```python
from build123d import *

# Parameters (mm, degrees)
BOSS_EXTRUDE1_DEPTH = 35.179
CUT_EXTRUDE2_START  = -5.0038
SKETCH2_R           = 4
CUT_EXTRUDE2_DEPTH  = 5.0038
CUT_EXTRUDE3_START  = -5.674182
CUT_EXTRUDE3_DEPTH  = 5.674182


with BuildPart() as part:
    # Sketch1 → Boss-Extrude1 (new, symmetric)
    with BuildSketch(Plane.XY):
        Polygon((0, 0), (27.178, 0), (27.178, 5.0038), (1.340764169, 5.0038), (-15.645662336, 14.810917915), (-18.147562336, 10.4775), align=None)
    extrude(amount=BOSS_EXTRUDE1_DEPTH, both=True)

    # Sketch2 → Cut-Extrude2 (cut)
    with BuildSketch(Plane.XZ.offset(CUT_EXTRUDE2_START)):
        with Locations(Location((13.462, 0, 0), (0, 0, 270))):
            Circle(SKETCH2_R)
        with BuildLine():
            Line((1.340764169, 35.179), (53.015235831, 35.179))
            Line((53.015235831, 35.179), (53.015235831, -35.179))
            Line((53.015235831, -35.179), (1.340764169, -35.179))
            ThreePointArc((1.340764169, -35.179), (8.255118058, -33.308689777), (13.28379292, -28.207829149))
            Line((13.28379292, -28.207829149), (25.405028751, -6.744829149))
            ThreePointArc((25.405028751, -6.744829149), (27.178, 0), (25.405028751, 6.744829149))
            Line((25.405028751, 6.744829149), (13.28379292, 28.207829149))
            ThreePointArc((13.28379292, 28.207829149), (8.255118058, 33.308689777), (1.340764169, 35.179))
        make_face()
    extrude(amount=CUT_EXTRUDE2_DEPTH, mode=Mode.SUBTRACT)

    # Sketch3 → Cut-Extrude3 (cut)
    with BuildSketch(Plane(origin=(0, 0, 0), x_dir=(0, 0, 1), z_dir=(-0.4999999999999947, -0.8660254037844417, 0)).offset(CUT_EXTRUDE3_START)):
        with BuildLine():
            Line((22.606, 6.928764169), (-22.606, 6.928764169))
            ThreePointArc((-22.606, 6.928764169), (-25.4, 4.134764169), (-22.606, 1.340764169))
            Line((-22.606, 1.340764169), (22.606, 1.340764169))
            ThreePointArc((22.606, 1.340764169), (25.4, 4.134764169), (22.606, 6.928764169))
        make_face()
        with BuildLine():
            Line((-35.179, -1.161135831), (-35.179, 43.071135831))
            Line((-35.179, 43.071135831), (35.179, 43.071135831))
            Line((35.179, 43.071135831), (35.179, -1.161135831))
            ThreePointArc((35.179, -1.161135831), (34.029362855, 4.335697857), (30.773170225, 8.911072784))
            ThreePointArc((30.773170225, 8.911072784), (0, 20.955), (-30.773170225, 8.911072784))
            ThreePointArc((-30.773170225, 8.911072784), (-34.029362855, 4.335697857), (-35.179, -1.161135831))
        make_face()
    extrude(amount=CUT_EXTRUDE3_DEPTH, mode=Mode.SUBTRACT)


solid = part.part
```
Check sheet for the modelled part. Datum: model origin and axes. Units: mm. A direction names the side the tool comes from. Round coordinates to 2 decimals unless told otherwise and drop trailing zeros. Loops run counter-clockwise (first coordinate to the right, second up) from the corner with the lowest first, then second, coordinate; pieces in that order, holes last. Notation, with made-up numbers: (62.5, -22.5) - (76.5, -22.5) arc R27 ccw to (76.5, 13.5) - close; hole circle Ø5 at (55.25, -6). An arc over 180 degrees is marked (long way). Write item = value, one per line. Start each with the question number.
Q1. Access from +Z, -Z, +X, -X, +Y, -Y to the whole of each face (thin tool, end or side, straight path). Record for faces 1 (the face through (-2.4, 4.3, -25.4)), 2 (the face through (0.11, 2.87, -0.32)), 3 (the face through (-7.034, 9.839, 0.489)).
Q2. Release check for a two-part mould opening along X. For faces 4 (the face through (8.34, 2.54, 33.26)), 5 (the face through (9, 5.004, 0)), 6 (the face through (-2.3, 4.2, 25.4)), 7 (the face through (-4.732, 5.661, 0.316)) record: pulls with the +X half, pulls with the -X half, needs draft (parallel to the pull), parting line crosses it, or undercut.
Q3. Thickness scan on L1, parallel to X at y = 3.9, z = 0 (3 decimals); L2, parallel to Y at x = 23, z = 1.5; L3, parallel to Z at x = 11, y = 2.5. Record the ranges inside material, lowest first.
Q4. Section check C-C (z = 19). Record the boundary of the cut face in (x, y).
Q5. Section check B-B (x = 14.5). Record the boundary of the cut face in (y, z).
Q6. Depth check by flat-ended pin: P1, Ø5, axis at y = 5, z = 24, coming from the -X side; P2, Ø5, axis at x = 5, y = 4, coming from the +Z side; P3, Ø1.5, axis at x = -5.5, y = 9, coming from the +Z side. Enter the tip coordinate at first touch or a pass-through.
Q7. Section check A-A (z = 0). Record the boundary of the cut face in (x, y), plus the area to 3 significant figures.
Derived:
q1.face_1 = none
q1.face_2 = +Y
q1.face_3 = +Z, -Z, +X, +Y
q2.face_4 = pulls with the +X half
q2.face_5 = needs draft
q2.face_6 = undercut
q2.face_7 = undercut
q3.L1 = -6.755 to -5.749, 0.703 to 9.462, 17.462 to 27.178
q3.L2 = 0 to 5
q3.L3 = -31.2 to -3.15, 3.15 to 31.2
q4.outline = (-14.53, 8.39) - (-6, 3.46) - (-3.5, 7.8) - (-12.03, 12.72) - close; (-1.16, 0.67) - (0, 0) - (18.48, 0) - (18.48, 5) - (1.34, 5) - close
q5.outline = (0, -26.05) - (5, -26.05) - (5, -3.86) - (0, -3.86) - close; (0, 3.86) - (5, 3.86) - (5, 26.05) - (0, 26.05) - close
q6.P1 = -12.68
q6.P2 = 35.13
q6.P3 = 31.18
q7.outline = (-18.15, 10.48) - (-6, 3.46) - (-3.5, 7.8) - (-15.65, 14.81) - close; (-1.16, 0.67) - (0, 0) - (9.46, 0) - (9.46, 5) - (1.34, 5) - close; (17.46, 0) - (27.18, 0) - (27.18, 5) - (17.46, 5) - close
q7.area = 166 mm^2
